Answer from the drawing. Dimensions are ordinates in mm from the lowest x, y and z of the part. Round coordinates to 2 decimals unless told otherwise and drop trailing zeros. Return JSON: item names as keys, results as strings. Group by question number.
(1) Straight lines are drawn through the part: line 1 (X direction, y = 11, z = 1) (1 decimal); line 2 (X direction, y = 25.5, z = 1.7); line 3 (X direction, y = 15.5, z = 2.1). For each, find the intervals that lie inside material, in ascending order.
(2) Given pin 1 (3 mm diameter, centred on x = 132.715, y = 20.955, fed in from +Z); pin 2 (1 mm diameter, centred on x = 245, z = 1, fed in from -Y), each flat-ended and moving along its own axis, determine where each tip first touches the part or whether it passes through.
(3) A cutting plane is placed at B-B on z = 1.05. State how many separate pieces and enclosed holes the cut face has, then the cut area to 3 significant figures.
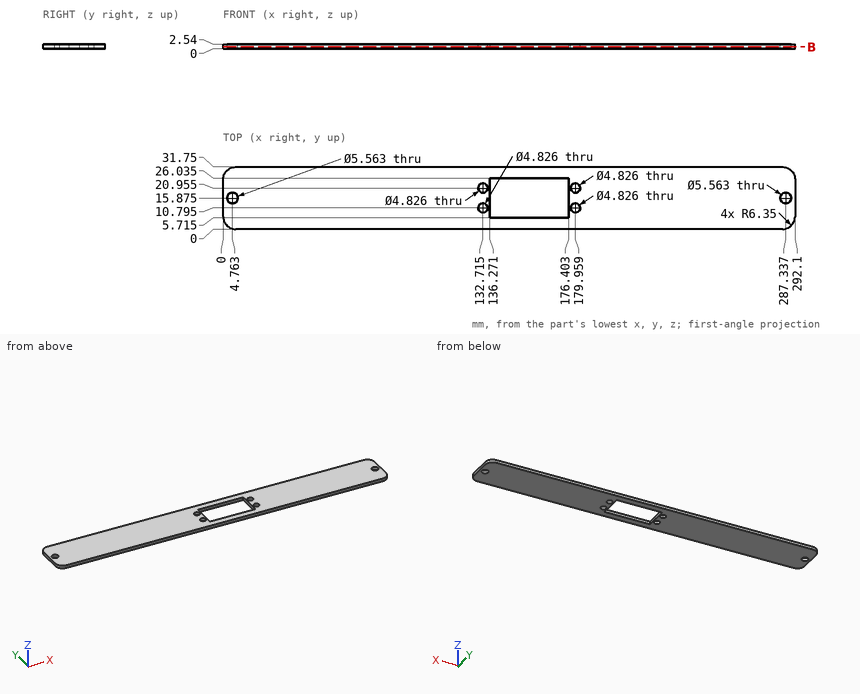
Checks:
{
 "1": {"line 1": "x = 0 to 130.3, 135.1 to 136.3, 176.4 to 177.6, 182.4 to 292.1", "line 2": "x = 0 to 136.27, 176.4 to 292.1", "line 3": "x = 0 to 2.01, 7.52 to 136.27, 176.4 to 284.58, 290.09 to 292.1"},
 "2": {"pin 1": "passes through", "pin 2": "stops at y = 0"},
 "3": {"separate pieces": "1", "enclosed holes": "7", "area": "8,300 mm^2"}
}
